Source: CAD feature listing. Evaluate the final solid. Frame: model axes, mm. Give positions to 0.01 mm unless a question says otherwise; leave off trailing zeros. Write each loop counter-clockwise with the first axis right and the second up, starting at its lowest first coordinate (ties: lowest second). Pieces come first, ordered by that corner, then holes. Notation, with made-up numbers: (4.5, 9) -> (49.5, 9) arc R29 cw to (49.5, 29) -> close; hole circle Ø1 at (-30, -20.5). An arc over 180 degrees is marked (long way). Answer as a JSON object with one key per item and string values. Group by question number.
Item 1: Pull-direction query (Z, two-part tool) for faces 1 (the face through (-81.16, 1.29, -26.5)), 2 (the face through (-75, 0, -20)), 3 (the face through (-77, 1, -50.8)); classes: pulls with the +Z half, pulls with the -Z half, needs draft (parallel to the pull), parting line crosses it, or undercut.
Item 2: Section query C-C on y = 0.4. Return the cut outline in (x, z).
Item 3: First-contact query: pin 1 Ø1 at (y, z) = (1, -34.5) entering from -X; pin 2 Ø1.5 at (y, z) = (0.5, -9) entering from -X (3 decimals). Flat tips, straight axial feed; report the tip coordinate or a pass-through.
Item 4: Section query D-D on x = -41.5. Return the cut outline in (y, z).
Item 5: Section query A-A on z = -25.4. Return the cut outline in (x, y), plus the area to 3 significant figures.
Item 6: Section query B-B on x = -76.2. Return the cut outline in (y, z), plus the area to 3 significant figures.
Item 7: Ray query, probe 1 along X at (y, z) = (1.7, -25.4); probe 2 along X at (y, z) = (0.45, -24); probe 3 along X at (y, z) = (2.3, -17.5). Return the intervals inside material, ascending. Write a range as from..to.
from build123d import *

# Parameters (mm, degrees)
BOSS_EXTRUDE1_DEPTH = 2.54
SKETCH2_R           = 5.08
CUT_EXTRUDE1_DEPTH  = 161.663784345


with BuildPart() as part:
    # Sketch1 → Boss-Extrude1 (new body)
    with BuildSketch(Plane(origin=(0, 0, 0), x_dir=(1, 0, 0), z_dir=(0, 1, 0))):
        Polygon((0, 0), (-152.4, 0), (-127, 50.8), (-25.4, 50.8), align=None)
    extrude(amount=BOSS_EXTRUDE1_DEPTH)

    # Sketch2 → Cut-Extrude1 (cut, through all)
    with BuildSketch(Plane(origin=(0, 2.54, 0), x_dir=(1, 0, 0), z_dir=(0, 1, 0))):
        with Locations(Location((-76.2, 25.4, 0), (0, 0, 270))):
            Circle(SKETCH2_R)
        with Locations(Location((-114.3, 25.4, 0), (0, 0, 270))):
            Circle(SKETCH2_R)
        with Locations(Location((-38.1, 25.4, 0), (0, 0, 270))):
            Circle(SKETCH2_R)
    extrude(amount=-CUT_EXTRUDE1_DEPTH, mode=Mode.SUBTRACT)


solid = part.part
Worked answers:
{
 "1": {"face 1": "undercut", "face 2": "needs draft", "face 3": "pulls with the -Z half"},
 "2": {"outline": "(-152.4, 0) -> (-127, -50.8) -> (-25.4, -50.8) -> (0, 0) -> close; hole circle Ø10.16 at (-114.3, -25.4); hole circle Ø10.16 at (-76.2, -25.4); hole circle Ø10.16 at (-38.1, -25.4)"},
 "3": {"pin 1": "x = -135.4", "pin 2": "x = -148.275"},
 "4": {"outline": "(0, -50.8) -> (2.54, -50.8) -> (2.54, -29.17) -> (0, -29.17) -> close; (0, -21.63) -> (2.54, -21.63) -> (2.54, 0) -> (0, 0) -> close"},
 "5": {"outline": "(-139.7, 0) -> (-119.38, 0) -> (-119.38, 2.54) -> (-139.7, 2.54) -> close; (-109.22, 0) -> (-81.28, 0) -> (-81.28, 2.54) -> (-109.22, 2.54) -> close; (-71.12, 0) -> (-43.18, 0) -> (-43.18, 2.54) -> (-71.12, 2.54) -> close; (-33.02, 0) -> (-12.7, 0) -> (-12.7, 2.54) -> (-33.02, 2.54) -> close", "area": "245 mm^2"},
 "6": {"outline": "(0, -50.8) -> (2.54, -50.8) -> (2.54, -30.48) -> (0, -30.48) -> close; (0, -20.32) -> (2.54, -20.32) -> (2.54, 0) -> (0, 0) -> close", "area": "103 mm^2"},
 "7": {"probe 1": "-139.7..-119.38, -109.22..-81.28, -71.12..-43.18, -33.02..-12.7", "probe 2": "-140.4..-119.18, -109.42..-81.08, -71.32..-42.98, -33.22..-12", "probe 3": "-143.65..-8.75"}
}
